Build history of the part. All positions in model axes, mm. A direction names the side the tool comes from. Round coordinates to 2 decimals unless told otherwise and drop trailing zeros. Write each loop counter-clockwise with the first axis right and the second up, starting at its lowest first coordinate (ties: lowest second). Pieces come first, ordered by that corner, then holes.
Item 1: Wall check: probe 1 along Y at (x, z) = (0, 41.5); probe 2 along Y at (x, z) = (792, 1365); probe 3 along Z at (x, y) = (162.5, -83.5). Give the ranges that are in metal, low to high.
Item 2: Band-saw the part on B-B, the plane z = 1658. Write the cut outline in (x, y).
Item 3: Band-saw the part on A-A, the plane x = 775. Write the cut outline in (y, z).
Item 4: Mould opens along X. For faces 5 (the flat face through (65, 4, 0)), 6 (the flat face through (849.065, -1.05, 879.28)), 7 (the cylindrical face through (1274.325, -1.05, 1833.431)) say: +X half, -X half, draft (parallel to the pull), parting line (faces both ways), or undercut.
Item 5: Drop flat-ended pins along their axis: pin 1 Ø10 at (x, z) = (-308.5, 7.5) entering from -Y; pin 2 Ø24.5 at (x, y) = (-33.5, 101.5) entering from +Z; pin 3 Ø7.5 at (x, z) = (-310, 8) entering from +Y. Give the stop position or say it passes through.
Item 6: 3-axis set-ups, long thin cutter, end or side, ignore diameter. For faces 1 (the flat face through (-2, -106, 187.5)), 2 (the cylindrical face through (1367.54, -1.05, 1949.84)), 3 (the flat face through (-2, 107, 187.5)), 4 (the cylindrical face through (-62.44, -2.75, 36.98)): which of +Z, -Z, +X, -X, +Y, -Y reach the whole face in a straight line?
Autodesk Fusion 360 part; units mm, degrees
sketch "Sketch1" plane through (0, 0, 0) normal (0, 0, 1) x (1, 0, 0)
  circle A0 centre (0, 0) radius 125
  dimension "d1" = 250
extrude "Extrude1" add sketch "Sketch1" along normal blind 75
fillet "Fillet1" radius 62.5 1 edges at (-116.5409, -45.2019, 75)
sketch "Sketch2" plane through (0, 0, 0) normal (0, 0, -1) x (1, 0, 0)
  circle A0 centre (0, 0) radius 125
  circle A1 centre (0, 0) radius 25
  dimension "d6" = 50
extrude "Extrude2" cut sketch "Sketch2" against normal blind 25 contours A1
sketch "Sketch3" plane through (0, 0, 0) normal (0, 1, 0) x (1, 0, 0)
  line L0 (62.5, -75) -> (-62.5, -75)
  line L1 (-125, 0) -> (125, 0)
  line L2 (-125, 0) -> (478.3021, -770.2875)
  line L3 (125, 0) -> (560.3465, -713.412)
  arc A0 (478.3021, -770.2875) -> (560.3465, -713.412) centre (517.6658, -739.4572) ccw
  circle A1 centre (517.6658, -739.4572) radius 10
  dimension "d23" = 100
  dimension "d24" = 20
extrude "Extrude6" add sketch "Sketch3" along normal blind 30 and the other way blind 30
sketch "Sketch5" plane through (0, 0, 0) normal (0, 0, -1) x (1, 0, 0)
  arc A0 (121.3466, 30) -> (-121.3466, 30) centre (0, 0) ccw
  line L0 (-121.3466, 30) -> (-125, 30)
  line L1 (-125, 30) -> (-125, 0)
  line L2 (-125, 0) -> (-125, -30)
  line L3 (-125, -30) -> (-121.3466, -30)
  arc A1 (-121.3466, -30) -> (121.3466, -30) centre (0, 0) ccw
  line L4 (121.3466, -30) -> (125, -30)
  line L5 (125, -30) -> (125, 30)
  line L6 (125, 30) -> (121.3466, 30)
  circle A2 centre (0, 0) radius 25
  dimension "d29" = 50
extrude "Extrude7" cut sketch "Sketch5" against normal blind 30 contours A2
scale "Scale1" factor 2.5 about (0, 0, 0) bodies 1
Results:
1. probe 1: y = -312.16 to -62.5, 62.5 to 312.16
1. probe 2: y = -75 to 75
1. probe 3: z = 0 to 185.25
2. outline: (986.07, -75) - (1324.26, -75) - (1324.26, 75) - (986.07, 75) - close
3. outline: (-75, 757.91) - (75, 757.91) - (75, 1388.5) - (-75, 1388.5) - close
4. face 5: draft
4. face 6: +X half
4. face 7: undercut
5. pin 1: stops at y = -75
5. pin 2: stops at z = 187.5
5. pin 3: stops at y = 75
6. face 1: +Z, +X, -X, -Y
6. face 2: +Y, -Y
6. face 3: +Z, +X, -X, +Y
6. face 4: -Z
